```python
from build123d import *

# Parameters (mm, degrees)
SKETCH_1_W          = 15
SKETCH_1_H          = 15
SKETCH_1_W_2        = 12
SKETCH_1_H_2        = 12
EXTRUDE_1_DEPTH     = 497.5
SKETCH_2_R          = 2.15
CUT_EXTRUDE_1_DEPTH = 498.782583062
SKETCH_3_R          = 2.15
CUT_EXTRUDE_2_DEPTH = 498.782583062


with BuildPart() as part:
    # ｽｹｯﾁ1 → 押し出し-薄板1 (new body)
    with BuildSketch(Plane(origin=(0, 0, 0), x_dir=(1, 0, 0), z_dir=(0, 1, 0))):
        Rectangle(SKETCH_1_W, SKETCH_1_H)
        Rectangle(SKETCH_1_W_2, SKETCH_1_H_2, mode=Mode.SUBTRACT)
    extrude(amount=EXTRUDE_1_DEPTH)

    # ｽｹｯﾁ2 → ｶｯﾄ - 押し出し1 (cut, through all)
    with BuildSketch(Plane(origin=(7.5, 0, 0), x_dir=(0, 0, -1), z_dir=(1, 0, 0))):
        with Locations((0, 71)):
            Circle(SKETCH_2_R)
        with Locations((0, 101)):
            Circle(SKETCH_2_R)
    extrude(amount=-CUT_EXTRUDE_1_DEPTH, mode=Mode.SUBTRACT)

    # ｽｹｯﾁ3 → ｶｯﾄ - 押し出し2 (cut, through all)
    with BuildSketch(Plane.XY.offset(7.5)):
        with Locations((0, 35)):
            Circle(SKETCH_3_R)
        with Locations((0, 5)):
            Circle(SKETCH_3_R)
        with Locations((0, 297.5)):
            Circle(SKETCH_3_R)
        with Locations((0, 327.5)):
            Circle(SKETCH_3_R)
        with Locations((0, 490)):
            Circle(SKETCH_3_R)
        with Locations((0, 460)):
            Circle(SKETCH_3_R)
    extrude(amount=-CUT_EXTRUDE_2_DEPTH, mode=Mode.SUBTRACT)


solid = part.part
```
Here's how the part is built. I have some questions about the finished solid (model axes, mm). A direction names the side the tool comes from. Coordinates: 2 decimals unless noted, no trailing zeros. Loops run counter-clockwise (first coordinate to the right, second up) from the corner with the lowest first, then second, coordinate; pieces in that order, holes last. Notation, with made-up numbers: (57, -20.5) -> (96, -20.5) arc R18 ccw to (96, -8.5) -> close; hole circle Ø2 at (-17, 51). An arc over 180 degrees is marked (long way). Return JSON: item names as keys, results as strings.
1) If we section it at A-A, the plane y = 145.5: Write out the boundary of the cut face in (x, z).
Results below:
{"outline": "(-7.5, -7.5) -> (7.5, -7.5) -> (7.5, 7.5) -> (-7.5, 7.5) -> close; hole (-6, -6) -> (6, -6) -> (6, 6) -> (-6, 6) -> close"}
2) For faces 1 (the face through (0, 245, -6)), 2 (the face through (-7, 0, 0)), which set-ups out of +Z, -Z, +X, -X, +Y, -Y let a thin tool reach every point of the face, with its end or its side?
Results below:
{"face 1": "+Y, -Y", "face 2": "+Z, -Z, +X, -X, -Y"}
3) Thinking about a two-plate mould opening in X: for faces 3 (the face through (6, 245, 0)), 4 (the face through (0, 245, 7.5)), 5 (the face through (-7.5, 245, 0)), which applies, +X half, -X half, draft (parallel to the pull), parting line (faces both ways), or undercut?
Results below:
{"face 3": "undercut", "face 4": "draft", "face 5": "-X half"}
4) I need wall thicknesses on line 1 (Y direction, x = -7, z = 0); line 2 (Z direction, x = 1.25, y = 198); line 3 (X direction, y = 297.5, z = 6.35). Which ranges of each line are inside material? Lowest first, please. Write a range as from..to.
Results below:
{"line 1": "0..68.85, 73.15..98.85, 103.15..497.5", "line 2": "-7.5..-6, 6..7.5", "line 3": "-7.5..-2.15, 2.15..7.5"}
